```python
from build123d import *

# Parameters (mm, degrees)
BASE_FLANGE1_DEPTH = 200
SKETCH6_R          = 1.5
CUT_EXTRUDE1_DEPTH = 10
SKETCH7_R          = 1.75
CUT_EXTRUDE2_DEPTH = 10
FILLET1_R          = 5
SKETCH8_R          = 1.5
CUT_EXTRUDE3_DEPTH = 10


# Read off the part's stored shape, not the designer's step: Base-Flange1
with BuildPart() as part:
    # Base-Flange1 outline → Base-Flange1 (new body)
    with BuildSketch(Plane.XY):
        with BuildLine():
            Line((-87.94, 48.076), (-87.94, 60))
            Line((-87.94, 60), (-90, 60))
            Line((-90, 60), (-90, 48.076))
            ThreePointArc((-90, 48.076), (-89.099060459, 45.900939541), (-86.924, 45))
            Line((-86.924, 45), (-1.016, 45))
            ThreePointArc((-1.016, 45), (-0.29757951, 44.70242049), (0, 43.984))
            Line((0, 43.984), (0, 3.076))
            ThreePointArc((0, 3.076), (0.900939541, 0.900939541), (3.076, 0))
            Line((3.076, 0), (15, 0))
            Line((15, 0), (15, 2.06))
            Line((15, 2.06), (3.076, 2.06))
            ThreePointArc((3.076, 2.06), (2.35757951, 2.35757951), (2.06, 3.076))
            Line((2.06, 3.076), (2.06, 43.984))
            ThreePointArc((2.06, 43.984), (1.159060459, 46.159060459), (-1.016, 47.06))
            Line((-1.016, 47.06), (-86.924, 47.06))
            ThreePointArc((-86.924, 47.06), (-87.64242049, 47.35757951), (-87.94, 48.076))
        make_face()
    extrude(amount=BASE_FLANGE1_DEPTH)

    # Sketch6 → Cut-Extrude1 (cut)
    with BuildSketch(Plane(origin=(-87.94, 0, 0), x_dir=(0, 0, -1), z_dir=(1, 0, 0))):
        with Locations((-190, 53.53)):
            Circle(SKETCH6_R)
        with Locations((-10, 53.53)):
            Circle(SKETCH6_R)
    extrude(amount=-CUT_EXTRUDE1_DEPTH, mode=Mode.SUBTRACT)

    # Sketch7 → Cut-Extrude2 (cut)
    with BuildSketch(Plane(origin=(0, 2.06, 0), x_dir=(1, 0, 0), z_dir=(0, 1, 0))):
        with Locations(Location((8.53, -10, 0), (0, 0, 270))):
            Circle(SKETCH7_R)
        with Locations(Location((8.53, -190, 0), (0, 0, 270))):
            Circle(SKETCH7_R)
    extrude(amount=-CUT_EXTRUDE2_DEPTH, mode=Mode.SUBTRACT)

    # Fillet1
    fillet1_edges = [part.edges().sort_by_distance(p)[0] for p in [
        (15, 1.03, 0),
        (-88.97, 60, 0),
        (15, 1.03, 200),
        (-88.97, 60, 200),
    ]]
    fillet(fillet1_edges, radius=FILLET1_R)

    # Sketch8 → Cut-Extrude3 (cut)
    with BuildSketch(Plane(origin=(0, 47.06, 0), x_dir=(1, 0, 0), z_dir=(0, 1, 0))):
        with Locations(Location((-82, -181.59, 0), (0, 0, 180))):
            Circle(SKETCH8_R)
        with Locations(Location((-48.35, -181.59, 0), (0, 0, 180))):
            Circle(SKETCH8_R)
        with Locations(Location((-48.35, -132.94, 0), (0, 0, 180))):
            Circle(SKETCH8_R)
        with Locations(Location((-82, -132.94, 0), (0, 0, 180))):
            Circle(SKETCH8_R)
        with Locations((-5.94, -132.94)):
            Circle(SKETCH8_R)
        with Locations((-39.59, -132.94)):
            Circle(SKETCH8_R)
        with Locations((-39.59, -181.59)):
            Circle(SKETCH8_R)
        with Locations((-5.94, -181.59)):
            Circle(SKETCH8_R)
        with Locations(Location((-5.94, -18.41, 0), (0, 0, 180))):
            Circle(SKETCH8_R)
        with Locations(Location((-39.59, -18.41, 0), (0, 0, 180))):
            Circle(SKETCH8_R)
        with Locations(Location((-39.59, -67.06, 0), (0, 0, 180))):
            Circle(SKETCH8_R)
        with Locations(Location((-5.94, -67.06, 0), (0, 0, 180))):
            Circle(SKETCH8_R)
        with Locations((-82, -67.06)):
            Circle(SKETCH8_R)
        with Locations((-48.35, -67.06)):
            Circle(SKETCH8_R)
        with Locations((-48.35, -18.41)):
            Circle(SKETCH8_R)
        with Locations((-82, -18.41)):
            Circle(SKETCH8_R)
        with BuildLine():
            Line((-82, -190.09), (-5.94, -190.09))
            ThreePointArc((-5.94, -190.09), (-4.44, -191.59), (-5.94, -193.09))
            Line((-5.94, -193.09), (-82, -193.09))
            ThreePointArc((-82, -193.09), (-83.5, -191.59), (-82, -190.09))
        make_face()
        with BuildLine():
            Line((-82, -9.91), (-5.94, -9.91))
            ThreePointArc((-5.94, -9.91), (-4.44, -8.41), (-5.94, -6.91))
            Line((-5.94, -6.91), (-82, -6.91))
            ThreePointArc((-82, -6.91), (-83.5, -8.41), (-82, -9.91))
        make_face()
        with BuildLine():
            Line((-82, -103.5), (-5.94, -103.5))
            ThreePointArc((-5.94, -103.5), (-4.44, -105), (-5.94, -106.5))
            Line((-5.94, -106.5), (-82, -106.5))
            ThreePointArc((-82, -106.5), (-83.5, -105), (-82, -103.5))
        make_face()
        with BuildLine():
            Line((-82, -96.5), (-5.94, -96.5))
            ThreePointArc((-5.94, -96.5), (-4.44, -95), (-5.94, -93.5))
            Line((-5.94, -93.5), (-82, -93.5))
            ThreePointArc((-82, -93.5), (-83.5, -95), (-82, -96.5))
        make_face()
    extrude(amount=-CUT_EXTRUDE3_DEPTH, mode=Mode.SUBTRACT)


solid = part.part
```
Here's how the part is built. I have some questions about the finished solid (model axes, mm). A direction names the side the tool comes from. Round coordinates to 2 decimals unless told otherwise and drop trailing zeros. Loops run counter-clockwise (first coordinate to the right, second up) from the corner with the lowest first, then second, coordinate; pieces in that order, holes last. Notation, with made-up numbers: (4.25, 59) -> (13.25, 59) arc R17 ccw to (13.25, 71) -> close; hole circle Ø11 at (-39, 47.5). An arc over 180 degrees is marked (long way). Answer as CSV lines item,"result". Start each with the question number.
1. Imagine slicing it at C-C on y = 39.5. Write out the boundary of the cut face in (x, z), plus the area to 3 significant figures.
2. For faces 1 (the face through (-45, 45, 99)), 2 (the face through (2.06, 23, 99)), 3 (the face through (13, 1, 1)), which set-ups out of +Z, -Z, +X, -X, +Y, -Y let a thin tool reach every point of the face, with its end or its side?
3. Imagine slicing it at A-A on x = -20. Write out the boundary of the cut face in (y, z).
4. I'm going to push flat-ended pins straight in: P1, Ø1.5, axis at y = 26.5, z = 117.5, coming from the +X side; P2, Ø4, axis at x = -82, z = 132.94, coming from the -Y side; P3, Ø1.5, axis at x = 0, z = 48.5, coming from the +Y side. Where does each tip first touch, or does it pass through?
5. I need wall thicknesses on probe 1 along Z at (x, y) = (-27, 46.5); probe 2 along X at (y, z) = (45.55, 132.94); probe 3 along Y at (x, z) = (-68, 178). Which ranges of each line are inside material? Lowest first, please. Write a range as from..to.
6. Imagine slicing it at B-B on z = 27. Write out the boundary of the cut face in (x, y).
Solution:
1,outline,"(0, 0) -> (2.06, 0) -> (2.06, 200) -> (0, 200) -> close"
1,area,"412 mm²"
2,face 1,"+Z, -Z, -X, -Y"
2,face 2,"+Z, -Z, +X, +Y"
2,face 3,"-Z, +X, +Y, -Y"
3,outline,"(45, 0) -> (47.06, 0) -> (47.06, 6.91) -> (45, 6.91) -> close; (45, 9.91) -> (47.06, 9.91) -> (47.06, 93.5) -> (45, 93.5) -> close; (45, 96.5) -> (47.06, 96.5) -> (47.06, 103.5) -> (45, 103.5) -> close; (45, 106.5) -> (47.06, 106.5) -> (47.06, 190.09) -> (45, 190.09) -> close; (45, 193.09) -> (47.06, 193.09) -> (47.06, 200) -> (45, 200) -> close"
4,P1,"x = 2.06"
4,P2,"y = 45"
4,P3,"y = 47.05"
5,probe 1,"0..6.91, 9.91..93.5, 96.5..103.5, 106.5..190.09, 193.09..200"
5,probe 2,"-88.68..-83.5, -80.5..-49.85, -46.85..-41.09, -38.09..-7.44, -4.44..1.63"
5,probe 3,"45..47.06"
6,outline,"(-90, 48.08) arc R3.08 ccw to (-86.92, 45) -> (-1.02, 45) arc R1.02 cw to (0, 43.98) -> (0, 3.08) arc R3.08 ccw to (3.08, 0) -> (15, 0) -> (15, 2.06) -> (3.08, 2.06) arc R1.02 cw to (2.06, 3.08) -> (2.06, 43.98) arc R3.08 ccw to (-1.02, 47.06) -> (-86.92, 47.06) arc R1.02 cw to (-87.94, 48.08) -> (-87.94, 60) -> (-90, 60) -> close"
